from build123d import *

# Parameters (mm, degrees)
BOSS_EXTRUDE1_DEPTH               = 10
FILLET1_R                         = 50
FILLET2_R                         = 50
CUT_EXTRUDE1_DEPTH                = 4
SKETCH6_R                         = 6.5
CUT_EXTRUDE2_DEPTH                = 89.160365244
SKETCH7_R                         = 14
CUT_EXTRUDE3_DEPTH                = 14
CHAMFER1_SIZE                     = 4
FILLET3_R                         = 5
TAP_DRILL_FOR_M10X1_25_TAP1_D     = 8.8
TAP_DRILL_FOR_M10X1_25_TAP1_DEPTH = 20
TAP_DRILL_FOR_M10X1_25_TAP1_TIP   = 4.4
CHAMFER2_SIZE                     = 1
FILLET4_R                         = 2


with BuildPart() as part:
    # Sketch2 → Boss-Extrude1 (new, symmetric)
    with BuildSketch(Plane.XY):
        with BuildLine():
            Line((16, 64.5), (30, 64.5))
            Line((30, 64.5), (30, 7.5))
            Line((30, 7.5), (46, -57.5))
            Line((46, -57.5), (46, -72.5))
            Line((46, -72.5), (-46, -72.5))
            Line((-46, -72.5), (-46, -57.5))
            Line((-46, -57.5), (-30, 7.5))
            Line((-30, 7.5), (-30, 64.5))
            Line((-30, 64.5), (-16, 64.5))
            ThreePointArc((-16, 64.5), (0, 72.5), (16, 64.5))
        make_face()
    extrude(amount=BOSS_EXTRUDE1_DEPTH, both=True)

    # Fillet1
    fillet1_edges = [part.edges().sort_by_distance(p)[0] for p in [
        (-30, 7.5, 0),
    ]]
    fillet(fillet1_edges, radius=FILLET1_R)

    # Fillet2
    fillet2_edges = [part.edges().sort_by_distance(p)[0] for p in [
        (30, 7.5, 0),
    ]]
    fillet(fillet2_edges, radius=FILLET2_R)

    # Sketch5 → Cut-Extrude1 (cut)
    with BuildSketch(Plane.XY.offset(10)):
        with BuildLine():
            Line((-19.797077506, -1.255831282), (-31.801048121, -50.021961906))
            ThreePointArc((-31.801048121, -50.021961906), (-31.433196909, -51.733678202), (-29.859018363, -52.5))
            Line((-29.859018363, -52.5), (29.859018363, -52.5))
            ThreePointArc((29.859018363, -52.5), (31.433196909, -51.733678202), (31.801048121, -50.021961906))
            Line((31.801048121, -50.021961906), (19.797077506, -1.255831282))
            ThreePointArc((19.797077506, -1.255831282), (18.450909046, 6.09947647), (18, 13.56334964))
            Line((18, 13.56334964), (18, 25.5))
            ThreePointArc((18, 25.5), (17.414213562, 26.914213562), (16, 27.5))
            Line((16, 27.5), (-16, 27.5))
            ThreePointArc((-16, 27.5), (-17.414213562, 26.914213562), (-18, 25.5))
            Line((-18, 25.5), (-18, 13.56334964))
            ThreePointArc((-18, 13.56334964), (-18.450909046, 6.09947647), (-19.797077506, -1.255831282))
        make_face()
    cut_extrude1 = extrude(amount=-CUT_EXTRUDE1_DEPTH, mode=Mode.SUBTRACT)

    # Mirror1: Cut-Extrude1 across plane
    add(cut_extrude1.mirror(Plane.XY), mode=Mode.SUBTRACT)

    # Sketch6 → Cut-Extrude2 (cut, through all)
    with BuildSketch(Plane.XY.offset(10)):
        with Locations((0, 52.5)):
            Circle(SKETCH6_R)
    extrude(amount=-CUT_EXTRUDE2_DEPTH, mode=Mode.SUBTRACT)

    # Sketch7 → Cut-Extrude3 (cut)
    with BuildSketch(Plane.XY.offset(10)):
        with Locations((0, 52.5)):
            Circle(SKETCH7_R)
    extrude(amount=-CUT_EXTRUDE3_DEPTH, mode=Mode.SUBTRACT)

    # Chamfer1
    chamfer1_edges = [part.edges().sort_by_distance(p)[0] for p in [
        (-30, 64.5, 0),
        (30, 64.5, 0),
    ]]
    chamfer(chamfer1_edges, length=CHAMFER1_SIZE)

    # Fillet3
    fillet3_edges = [part.edges().sort_by_distance(p)[0] for p in [
        (-16, 64.5, 0),
        (16, 64.5, 0),
    ]]
    fillet(fillet3_edges, radius=FILLET3_R)

    # Tap Drill for M10x1.25 Tap1
    with Locations(Plane(origin=(0, -72.5, 0), x_dir=(-1, 0, 0), z_dir=(0, -1, 0))):
        with Locations((30, 0), (-30, 0)):
            Hole(TAP_DRILL_FOR_M10X1_25_TAP1_D / 2, depth=TAP_DRILL_FOR_M10X1_25_TAP1_DEPTH)
            with Locations((0, 0, -(TAP_DRILL_FOR_M10X1_25_TAP1_DEPTH + TAP_DRILL_FOR_M10X1_25_TAP1_TIP / 2))):  # 90° drill point
                Cone(0, TAP_DRILL_FOR_M10X1_25_TAP1_D / 2, TAP_DRILL_FOR_M10X1_25_TAP1_TIP, mode=Mode.SUBTRACT)

    # Chamfer2
    chamfer2_edges = [part.edges().sort_by_distance(p)[0] for p in [
        (-14, 52.5, 10),
    ]]
    chamfer(chamfer2_edges, length=CHAMFER2_SIZE)

    # Fillet4
    fillet4_edges = [part.edges().sort_by_distance(p)[0] for p in [
        (31.433196909, -51.733678202, 6),
        (0, -52.5, 6),
        (-31.433196909, -51.733678202, 6),
        (-25.799062814, -25.638896594, 6),
        (-18.450909046, 6.09947647, 6),
        (-18, 19.53167482, 6),
        (-17.414213562, 26.914213562, 6),
        (0, 27.5, 6),
        (17.414213562, 26.914213562, 6),
        (18, 19.53167482, 6),
        (18.450909046, 6.09947647, 6),
        (25.799062814, -25.638896594, 6),
        (31.433196909, -51.733678202, -6),
        (25.799062814, -25.638896594, -6),
        (18.450909046, 6.09947647, -6),
        (18, 19.53167482, -6),
        (17.414213562, 26.914213562, -6),
        (0, 27.5, -6),
        (-17.414213562, 26.914213562, -6),
        (-18, 19.53167482, -6),
        (-18.450909046, 6.09947647, -6),
        (-25.799062814, -25.638896594, -6),
        (-31.433196909, -51.733678202, -6),
        (0, -52.5, -6),
    ]]
    fillet(fillet4_edges, radius=FILLET4_R)


solid = part.part
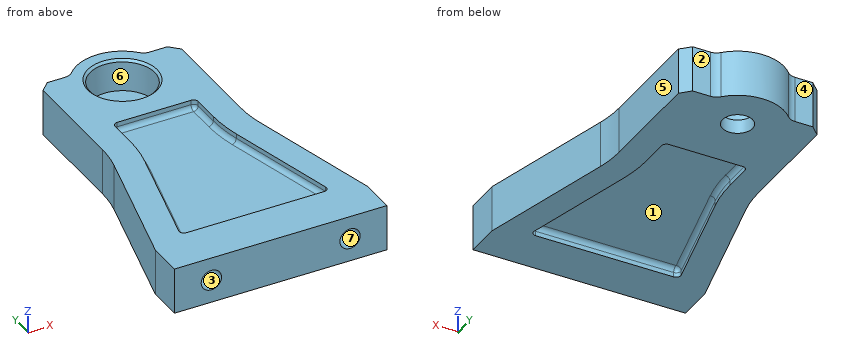
Here's how the part is built. I have some questions about the finished solid (model axes, mm). Face numbers are marked on the shaded views. A direction names the side the tool comes from. Coordinates: 2 decimals unless noted, no trailing zeros. Write each loop counter-clockwise with the first axis right and the second up, starting at its lowest first coordinate (ties: lowest second). Pieces come first, ordered by that corner, then holes.
1) If I drill on line 1 (Y direction, x = 0, z = 4.75); line 2 (Y direction, x = 0, z = -8.4); line 3 (Y direction, x = 0, z = -6.6), over which ranges is the centre line in solid material (lowest first)?
Filled in:
line 1: y = -72.5 to 38.5, 66.5 to 72.5
line 2: y = -72.5 to -52.5, 27.5 to 46, 59 to 72.5
line 3: y = -72.5 to -51.93, 26.93 to 46, 59 to 72.5
2) I'm going to push flat-ended pins straight in: pin 1 (5 mm diameter, centred on y = 48, z = 7.5, fed in from +X); pin 2 (1.5 mm diameter, centred on y = -15, z = -1.5, fed in from -X); pin 3 (5.5 mm diameter, centred on x = 30, z = 0, fed in from -Y). Where does each tip first touch, or does it pass through?
Filled in:
pin 1: stops at x = 30
pin 2: stops at x = -35.72
pin 3: stops at y = -50.85
3) If we section it at B-B (y = 52.5): List the corners of the cut face in (x, z) for me.
Filled in:
outline: (-30, -10) - (-6.5, -10) - (-6.5, -4) - (-14, -4) - (-14, 9) - (-15, 10) - (-30, 10) - close; (6.5, -10) - (30, -10) - (30, 10) - (15, 10) - (14, 9) - (14, -4) - (6.5, -4) - close
4) If we section it at A-A (x = 0): List the corners of the cut face in (y, z) for me, plus the area to 3 significant figures.
Filled in:
outline: (-72.5, -10) - (-52.5, -10) - (-52.5, -8) arc R2 cw to (-50.5, -6) - (25.5, -6) arc R2 cw to (27.5, -8) - (27.5, -10) - (46, -10) - (46, -4) - (38.5, -4) - (38.5, 9) - (37.5, 10) - (27.5, 10) - (27.5, 8) arc R2 cw to (25.5, 6) - (-50.5, 6) arc R2 cw to (-52.5, 8) - (-52.5, 10) - (-72.5, 10) - close; (59, -10) - (72.5, -10) - (72.5, 10) - (67.5, 10) - (66.5, 9) - (66.5, -4) - (59, -4) - close
area: 1,790 mm2
5) Thinking about a two-plate mould opening in Y: for the marked faces 1, 2 and 3, which applies, +Y half, -Y half, draft (parallel to the pull), parting line (faces both ways), or undercut?
Filled in:
face 1: undercut
face 2: +Y half
face 3: draft
6) Which directions (+Z, -Z, +X, -X, +Y, -Y) give clear straight access to the entire face, cutting with the end or side of a thin tool? Please do the marked faces 4, 5, 6 and 7.
Filled in:
face 4: +Z, -Z, -X, +Y
face 5: +Z, -Z, +X, +Y
face 6: +Z
face 7: -Y
